CAD build for the part. Positions are in the model's coordinates, mm. A direction names the side the tool comes from. Give positions to 0.01 mm unless a question says otherwise; leave off trailing zeros. Write each loop counter-clockwise with the first axis right and the second up, starting at its lowest first coordinate (ties: lowest second). Pieces come first, ordered by that corner, then holes. Notation, with made-up numbers: (56, -15.5) -> (103, -15.5) arc R16 ccw to (103, -11.5) -> close; hole circle Ø3 at (-35, 77). An arc over 180 degrees is marked (long way). Answer as a JSON object with one key per item and string values.
Autodesk Inventor part; units mm, degrees
ref_plane "YZ Plane" through (0, 0, 0) normal (1, 0, 0) x (0, 1, 0)
ref_plane "XZ Plane" through (0, 0, 0) normal (0, 1, 0) x (-1, 0, 0)
ref_plane "XY Plane" through (0, 0, 0) normal (0, 0, 1) x (1, 0, 0)
sketch "Sketch1" plane through (0, 0, 0) normal (1, 0, 0) x (0, 1, 0)
  line L0 (0, 29) -> (103.5, 29)
  line L1 (103.5, -29) -> (0, -29)
  line L2 (0, -29) -> (0, 29)
  line L3 (103.5, 29) -> (103.5, 26.5)
  line L4 (103.5, 26.5) -> (3, 26.5)
  line L5 (3, 26.5) -> (3, -26.5)
  line L6 (3, -26.5) -> (103.5, -26.5)
  line L7 (103.5, -26.5) -> (103.5, -29)
  point P0 (0, 0)
  point P1 (0, 0)
  dimension "d0" = 103.5
  dimension "d1" = 58
  dimension "d2" = 2.5
  dimension "d3" = 2.5
  dimension "d4" = 3
extrude "Extrusion1" add sketch "Sketch1" along normal blind 5.5
sketch "Sketch2" plane through (5.5, 0, 0) normal (1, 0, 0) x (0, 0, -1)
  circle A0 centre (39, 51.75) radius 2.5
  circle A1 centre (-39, 77.63) radius 2.5
  circle A2 centre (-39, 25.88) radius 2.5
  arc A3 (39, 41.75) -> (39, 61.75) centre (39, 51.75) ccw
  arc A4 (-39, 87.63) -> (-39, 67.63) centre (-39, 77.63) ccw
  arc A5 (-39, 35.88) -> (-39, 15.88) centre (-39, 25.88) ccw
  line L0 (-39, 87.63) -> (-29, 87.63)
  line L1 (-29, 87.63) -> (-29, 67.63)
  line L2 (-29, 67.63) -> (-39, 67.63)
  line L3 (-39, 35.88) -> (-29, 35.88)
  line L4 (-29, 35.88) -> (-29, 15.88)
  line L5 (-29, 15.88) -> (-39, 15.88)
  line L6 (39, 41.75) -> (29, 41.75)
  line L7 (29, 41.75) -> (29, 61.75)
  line L8 (29, 61.75) -> (39, 61.75)
  point P0 (0, 0)
  point P1 (-29, 0)
  point P2 (29, 0)
  dimension "d9" = 5
  dimension "d10" = 10
  dimension "d11" = 10
  dimension "d12" = 41.75
  dimension "d13" = 15.88
  dimension "d14" = 51.75
extrude "Extrusion2" add sketch "Sketch2" against normal blind 5.5
sketch "Sketch3" plane through (5.5, 0, 0) normal (1, 0, 0) x (0, 0, -1)
  line L0 (-27.5, 103.5) -> (27.5, 103.5)
  line L1 (27.5, 103.5) -> (27.5, 1.5)
  line L2 (27.5, 1.5) -> (-27.5, 1.5)
  line L3 (-27.5, 1.5) -> (-27.5, 103.5)
  line L4 (-26.5, 3) -> (-26.5, 103.5)
  line L5 (26.5, 103.5) -> (26.5, 3)
  line L6 (26.5, 3) -> (-26.5, 3)
  point P0 (0, 0)
  point P1 (-29, 103.5)
  dimension "d17" = 1
  dimension "d18" = 1
  dimension "d19" = 1.5
extrude "Extrusion3" cut sketch "Sketch3" against normal blind 3.5
equation "\"d3\" = d2"
equation "\"d18\" = d17"
properties material "ABS Plastic"
1) Slice it at D-D (z = 15.5). List the corners of the cut face in (x, y), then the cut area to 4 significant figures.
Model answer:
{"outline": "(0, 0) -> (5.5, 0) -> (5.5, 1.5) -> (2, 1.5) -> (2, 3) -> (0, 3) -> close", "area": "11.25 mm2"}
2) Slice it at C-C (y = 11). List the corners of the cut face in (x, z).
Model answer:
{"outline": "(0, -29) -> (5.5, -29) -> (5.5, -27.5) -> (2, -27.5) -> (2, -26.5) -> (0, -26.5) -> close; (0, 26.5) -> (2, 26.5) -> (2, 27.5) -> (5.5, 27.5) -> (5.5, 29) -> (0, 29) -> close"}
3) Slice it at A-A (y = 51.75). List the corners of the cut face in (x, z), then the cut area to 3 significant figures.
Model answer:
{"outline": "(0, -49) -> (5.5, -49) -> (5.5, -41.5) -> (0, -41.5) -> close; (0, -36.5) -> (5.5, -36.5) -> (5.5, -27.5) -> (2, -27.5) -> (2, -26.5) -> (0, -26.5) -> close; (0, 26.5) -> (2, 26.5) -> (2, 27.5) -> (5.5, 27.5) -> (5.5, 29) -> (0, 29) -> close", "area": "103 mm2"}
4) Mould opens along Z. For faces 1 (the cylindrical face through (2.788, 51.53, -48.998)), 2 (the flat face through (3, 52, 29)), 3 (the cylindrical face through (2.79, 50.79, -41.31)) say: released by +Z, released by -Z, zero draft, split by the parting line, or undercut.
Model answer:
{"face 1": "released by -Z", "face 2": "released by +Z", "face 3": "undercut"}
5) Pin check, flat tips, straight feed: pin 1 (2 mm diameter, centred on x = 1, z = -30.5, fed in from +Y); pin 2 (3 mm diameter, centred on x = 4, z = 36.5, fed in from +Y); pin 3 (8 mm diameter, centred on y = 86.5, z = 24.5, fed in from -X); pin 4 (2 mm diameter, centred on x = 1, y = 56.5, fed in from +Z). Stop position of each tip, or through.
Model answer:
{"pin 1": "stops at y = 61.75", "pin 2": "stops at y = 87.63", "pin 3": "stops at x = 0", "pin 4": "stops at z = 29"}
6) Wall check: probe 1 along Y at (x, z) = (2.15, 39); probe 2 along Z at (x, y) = (1.15, 10.5); probe 3 along Z at (x, y) = (2.55, 9.5). Give the ranges that are in metal, low to high.
Model answer:
{"probe 1": "y = 15.88 to 23.38, 28.38 to 35.88, 67.63 to 75.13, 80.13 to 87.63", "probe 2": "z = -29 to -26.5, 26.5 to 29", "probe 3": "z = -29 to -27.5, 27.5 to 29"}
7) Slice it at B-B (x = 3.2). List the corners of the cut face in (y, z), then the cut area to 3 significant figures.
Model answer:
{"outline": "(0, -29) -> (41.75, -29) -> (41.75, -39) arc R10 ccw to (61.75, -39) -> (61.75, -29) -> (103.5, -29) -> (103.5, -27.5) -> (1.5, -27.5) -> (1.5, 27.5) -> (103.5, 27.5) -> (103.5, 29) -> (87.63, 29) -> (87.63, 39) arc R10 ccw to (67.63, 39) -> (67.63, 29) -> (35.88, 29) -> (35.88, 39) arc R10 ccw to (15.88, 39) -> (15.88, 29) -> (0, 29) -> close; hole circle Ø5 at (25.88, 39); hole circle Ø5 at (51.75, -39); hole circle Ø5 at (77.63, 39)", "area": "1,410 mm2"}
8) 3-axis set-ups, long thin cutter, end or side, ignore diameter. For faces 4 (the flat face through (2, 53, 27)), 5 (the cylindrical face through (2.79, 27.99, 37.66)), 6 (the flat face through (3, 21, -29)), 7 (the flat face through (3, 83, -29)), 8 (the flat face through (3, 8, 29)): which of +Z, -Z, +X, -X, +Y, -Y reach the whole face in a straight line?
Model answer:
{"face 4": "+X, +Y", "face 5": "+X, -X", "face 6": "-Z, +X, -X, -Y", "face 7": "-Z, +X, -X, +Y", "face 8": "+Z, +X, -X, -Y"}
